```python
from build123d import *

# Parameters (mm, degrees)
EXTRUDE_1_DEPTH     = 4
SKETCH_3_W          = 40.4
SKETCH_3_H          = 4.4
CUT_EXTRUDE_1_DEPTH = 510.640069068


with BuildPart() as part:
    # Эскиз1 → Бобышка-Вытянуть1 (new body)
    with BuildSketch(Plane(origin=(0, 0, 0), x_dir=(1, 0, 0), z_dir=(0, 1, 0))):
        Polygon((0, 0), (0, 20), (-4, 20), (-4, 50), (0, 50), (0, 70), (-4, 70), (-4, 100), (0, 100), (0, 120), (-4, 120), (-4, 150), (0, 150), (0, 170), (45, 170), (45, 174), (85, 174), (85, 170), (125, 170), (125, 174), (165, 174), (165, 170), (205, 170), (205, 174), (245, 174), (245, 170), (285, 170), (285, 174), (325, 174), (325, 170), (365, 170), (365, 174), (405, 174), (405, 170), (475, 170), (475, 150), (479, 150), (479, 120), (475, 120), (475, 100), (479, 100), (479, 70), (475, 70), (475, 50), (479, 50), (479, 20), (475, 20), (475, 0), (405, 0), (405, -4), (365, -4), (365, 0), (325, 0), (325, -4), (285, -4), (285, 0), (245, 0), (245, -4), (205, -4), (205, 0), (165, 0), (165, -4), (125, -4), (125, 0), (85, 0), (85, -4), (45, -4), (45, 0), align=None)
    extrude(amount=-EXTRUDE_1_DEPTH)

    # Эскиз3 → Вырез-Вытянуть1 (cut, through all)
    with BuildSketch(Plane(origin=(0, 0, 0), x_dir=(1, 0, 0), z_dir=(0, 1, 0))):
        with Locations((147.5, 27)):
            Rectangle(SKETCH_3_W, SKETCH_3_H)
        with Locations((327.5, 27)):
            Rectangle(SKETCH_3_W, SKETCH_3_H)
        with Locations((147.5, 56)):
            Rectangle(SKETCH_3_W, SKETCH_3_H)
        with Locations((327.5, 56)):
            Rectangle(SKETCH_3_W, SKETCH_3_H)
        with Locations((147.5, 85)):
            Rectangle(SKETCH_3_W, SKETCH_3_H)
        with Locations((327.5, 85)):
            Rectangle(SKETCH_3_W, SKETCH_3_H)
        with Locations((147.5, 114)):
            Rectangle(SKETCH_3_W, SKETCH_3_H)
        with Locations((327.5, 114)):
            Rectangle(SKETCH_3_W, SKETCH_3_H)
        with Locations((147.5, 143)):
            Rectangle(SKETCH_3_W, SKETCH_3_H)
        with Locations((327.5, 143)):
            Rectangle(SKETCH_3_W, SKETCH_3_H)
    extrude(amount=-CUT_EXTRUDE_1_DEPTH, mode=Mode.SUBTRACT)


solid = part.part
```
Check sheet for the modelled part. Datum: model origin and axes. Units: mm. Give positions to 0.01 mm unless a question says otherwise; leave off trailing zeros. Loops run counter-clockwise (first coordinate to the right, second up) from the corner with the lowest first, then second, coordinate; pieces in that order, holes last. Notation, with made-up numbers: (61.5, -26.5) - (93.5, -26.5) arc R30 ccw to (93.5, 4.5) - close; hole circle Ø11 at (55, -6.75). An arc over 180 degrees is marked (long way). One line per question, with ' | ' between items. Start each with the question number.
1. Cross-section at C-C, the plane y = -1. Give the number of separate pieces and of enclosed holes in the cut face, plus the area to 3 significant figures.
2. Cross-section at D-D, the plane x = 178. Enter the section's corners in (y, z), plus the area to 3 significant figures.
3. Gauge pin test, flat ends, axial feed: pin 1 Ø1 at (y, z) = (-3.5, -57) entering from -X; pin 2 Ø1.2 at (x, y) = (331, -2) entering from -Z; pin 3 Ø1 at (x, y) = (86.5, -1.5) entering from +Z. Record the tip position at first contact, or that the pin passes through.
4. Material ranges on line 1 along Z through (x, y) = (333.5, -2.15); line 2 along X through (y, z) = (-1.85, -54); line 3 along Z through (x, y) = (177, -2.15), recorded low to high. Write a range as [from, to].
5. Cross-section at A-A, the plane x = 317. Enter the section's corners in (y, z), plus the area to 3 significant figures.
6. Cross-section at B-B, the plane z = -63. Enter the section's corners in (x, y), plus the area to 3 significant figures.
Check result:
1) separate pieces: 1 | enclosed holes: 10 | area: 81,300 mm2
2) outline: (-4, -170) - (0, -170) - (0, 0) - (-4, 0) - close | area: 680 mm2
3) pin 1: stops at x = 0 | pin 2: stops at z = -170 | pin 3: stops at z = 0
4) line 1: z = [-170, -145.2], [-140.8, -116.2], [-111.8, -87.2], [-82.8, -58.2], [-53.8, -29.2], [-24.8, 0] | line 2: x = [0, 127.3], [167.7, 307.3], [347.7, 475] | line 3: z = [-170, 0]
5) outline: (-4, -174) - (0, -174) - (0, -145.2) - (-4, -145.2) - close; (-4, -140.8) - (0, -140.8) - (0, -116.2) - (-4, -116.2) - close; (-4, -111.8) - (0, -111.8) - (0, -87.2) - (-4, -87.2) - close; (-4, -82.8) - (0, -82.8) - (0, -58.2) - (-4, -58.2) - close; (-4, -53.8) - (0, -53.8) - (0, -29.2) - (-4, -29.2) - close; (-4, -24.8) - (0, -24.8) - (0, 4) - (-4, 4) - close | area: 624 mm2
6) outline: (0, -4) - (475, -4) - (475, 0) - (0, 0) - close | area: 1,900 mm2
